Source: CAD feature listing. Evaluate the final solid. Frame: model axes, mm. A direction names the side the tool comes from. Give positions to 0.01 mm unless a question says otherwise; leave off trailing zeros. Loops run counter-clockwise (first coordinate to the right, second up) from the corner with the lowest first, then second, coordinate; pieces in that order, holes last.
```python
from build123d import *

# Parameters (mm, degrees)
SKETCH1_R           = 5.1
SKETCH1_R_2         = 1.25
SKETCH1_R_3         = 1.5
BOSS_EXTRUDE1_DEPTH = 3
FILLET1_R           = 3
CUT_EXTRUDE1_DEPTH  = 10
BOSS_EXTRUDE2_DEPTH = 3
CUT_EXTRUDE2_DEPTH  = 10
FILLET2_R           = 10


with BuildPart() as part:
    # Sketch1 → Boss-Extrude1 (new body)
    with BuildSketch(Plane(origin=(0, 0, 0), x_dir=(1, 0, 0), z_dir=(0, 1, 0))):
        with BuildLine():
            Line((70, 20), (-70, 20))
            ThreePointArc((-70, 20), (-90, 0), (-70, -20))
            Line((-70, -20), (-41, -20))
            Line((-41, -20), (-28.75, -7.75))
            Line((-28.75, -7.75), (-16.5, -20))
            Line((-16.5, -20), (70, -20))
            ThreePointArc((70, -20), (90, 0), (70, 20))
        make_face()
        with Locations(Location((70, 0, 0), (0, 0, 270))):
            Circle(SKETCH1_R, mode=Mode.SUBTRACT)
        with Locations(Location((59.837325142, 4.209517756, 0), (0, 0, 270))):
            Circle(SKETCH1_R_2, mode=Mode.SUBTRACT)
        with Locations(Location((65.790482244, 10.162674858, 0), (0, 0, 270))):
            Circle(SKETCH1_R_2, mode=Mode.SUBTRACT)
        with Locations(Location((74.209517756, 10.162674858, 0), (0, 0, 270))):
            Circle(SKETCH1_R_2, mode=Mode.SUBTRACT)
        with Locations(Location((80.162674858, 4.209517756, 0), (0, 0, 270))):
            Circle(SKETCH1_R_2, mode=Mode.SUBTRACT)
        with Locations(Location((80.162674858, -4.209517756, 0), (0, 0, 270))):
            Circle(SKETCH1_R_2, mode=Mode.SUBTRACT)
        with Locations(Location((74.209517756, -10.162674858, 0), (0, 0, 270))):
            Circle(SKETCH1_R_2, mode=Mode.SUBTRACT)
        with Locations(Location((65.790482244, -10.162674858, 0), (0, 0, 270))):
            Circle(SKETCH1_R_2, mode=Mode.SUBTRACT)
        with Locations(Location((59.837325142, -4.209517756, 0), (0, 0, 270))):
            Circle(SKETCH1_R_2, mode=Mode.SUBTRACT)
        with Locations(Location((-59.837325142, -4.209517756, 0), (0, 0, 90))):
            Circle(SKETCH1_R_2, mode=Mode.SUBTRACT)
        with Locations(Location((-65.790482244, -10.162674858, 0), (0, 0, 90))):
            Circle(SKETCH1_R_2, mode=Mode.SUBTRACT)
        with Locations(Location((-74.209517756, -10.162674858, 0), (0, 0, 90))):
            Circle(SKETCH1_R_2, mode=Mode.SUBTRACT)
        with Locations(Location((-80.162674858, -4.209517756, 0), (0, 0, 90))):
            Circle(SKETCH1_R_2, mode=Mode.SUBTRACT)
        with Locations(Location((-80.162674858, 4.209517756, 0), (0, 0, 90))):
            Circle(SKETCH1_R_2, mode=Mode.SUBTRACT)
        with Locations(Location((-74.209517756, 10.162674858, 0), (0, 0, 90))):
            Circle(SKETCH1_R_2, mode=Mode.SUBTRACT)
        with Locations(Location((-65.790482244, 10.162674858, 0), (0, 0, 90))):
            Circle(SKETCH1_R_2, mode=Mode.SUBTRACT)
        with Locations(Location((-59.837325142, 4.209517756, 0), (0, 0, 90))):
            Circle(SKETCH1_R_2, mode=Mode.SUBTRACT)
        with Locations(Location((-70, 0, 0), (0, 0, 90))):
            Circle(SKETCH1_R, mode=Mode.SUBTRACT)
        with Locations(Location((-35, 0, 0), (0, 0, 270))):
            Circle(SKETCH1_R_3, mode=Mode.SUBTRACT)
        with Locations(Location((-18.029437252, 16.970562748, 0), (0, 0, 270))):
            Circle(SKETCH1_R_3, mode=Mode.SUBTRACT)
    extrude(amount=BOSS_EXTRUDE1_DEPTH)

    # Fillet1
    fillet1_edges = [part.edges().sort_by_distance(p)[0] for p in [
        (-16.5, 1.5, 20),
        (-28.75, 1.5, 7.75),
        (-41, 1.5, 20),
    ]]
    fillet(fillet1_edges, radius=FILLET1_R)

    # Sketch2 → Cut-Extrude1 (cut)
    with BuildSketch(Plane.XZ):
        Polygon((-28.358163655, 9.01834005), (55, 20), (-28.358163655, 26.558419641), align=None)
    extrude(amount=-CUT_EXTRUDE1_DEPTH, mode=Mode.SUBTRACT)

    # Sketch3 → Boss-Extrude2 (add)
    with BuildSketch(Plane.XZ):
        Polygon((-70, -20), (-29.714195297, -26), (60, -20), align=None)
    extrude(amount=-BOSS_EXTRUDE2_DEPTH)

    # Sketch4 → Cut-Extrude2 (cut)
    with BuildSketch(Plane.XZ):
        Polygon((-29.761678485, 9.168369694), (-60, 20), (-60.52961588, 25.578691215), (-29.998372271, 24.401767037), align=None)
    extrude(amount=-CUT_EXTRUDE2_DEPTH, mode=Mode.SUBTRACT)

    # Fillet2
    # the kernel refuses this fillet: 10 mm, written as the material it adds along each edge
    with BuildSketch(Plane(origin=(60, 0, -20), x_dir=(-0.9977710708464071, 0, -0.06672997963445026), z_dir=(0, 1, 0))) as fillet2_piece_1:
        with BuildLine():
            CenterArc((FILLET2_R * 0.0334022154031, -FILLET2_R), FILLET2_R, 90, 3.826189391)
            Line((-FILLET2_R * 0.0333277642314, -FILLET2_R * 0.00222892915359), (0, 0))
            Line((0, 0), (FILLET2_R * 0.0334022154031, 0))
        make_face()
    extrude(amount=3)
    # the kernel refuses this fillet: 10 mm, written as the material it takes off along each edge
    with BuildSketch(Plane(origin=(-29.714195297, -2.693204599, -26), x_dir=(-0.9890902260552777, 0, 0.14731097963804135), z_dir=(0, 1, 0))) as fillet2_2_piece_1:
        with BuildLine():
            CenterArc((FILLET2_R * 0.107728183948, FILLET2_R), FILLET2_R, 257.702684713, 12.297315287)
            Line((-FILLET2_R * 0.105256420594, FILLET2_R * 0.0229444446563), (0, 0))
            Line((0, 0), (FILLET2_R * 0.107728183948, 0))
        make_face()
    extrude(amount=8.386409197, mode=Mode.SUBTRACT)


solid = part.part
```
(1) Section A-A, the plane z = 0. Return the cut outline in (x, y).
A:
outline: (-90, 0) - (-75.1, 0) - (-75.1, 3) - (-90, 3) - close; (-64.9, 0) - (-36.5, 0) - (-36.5, 3) - (-64.9, 3) - close; (-33.5, 0) - (64.9, 0) - (64.9, 3) - (-33.5, 3) - close; (75.1, 0) - (90, 0) - (90, 3) - (75.1, 3) - close
(2) Ray query, line 1 along Z through (x, y) = (64.5, 2.4); line 2 along X through (y, z) = (1, 8.5); line 3 along X through (y, z) = (2.3, 8). Return the intervals inside material, ascending.
A:
line 1: z = -20 to 20
line 2: x = -88.1 to 88.1
line 3: x = -88.33 to 88.33
(3) Section B-B, the plane y = 0.7. Count the separate pieces of the cut face and the enclosed holes in it, then the cut area to 3 significant figures.
A:
separate pieces: 1
enclosed holes: 20
area: 6,350 mm2
(4) First-contact query: pin 1 (3 mm diameter, centred on x = -59.84, z = -4.21, fed in from +Y); pin 2 (1.8 mm diameter, centred on x = -35, z = 0, fed in from +Y); pin 3 (1 mm diameter, centred on y = 0.5, z = -5, fed in from +X). Flat tips, straight axial feed; report the tip coordinate or a pass-through.
A:
pin 1: stops at y = 3
pin 2: passes through
pin 3: stops at x = 89.49
(5) Reachability of faces 1 (the flat face through (-44.67, 1.48, 14.51)), 2 (the cylindrical face through (-75, 1, 1)), 3 (the flat face through (65, 1, -20)) from +Z, -Z, +X, -X, +Y, -Y: full face, straight path, thin tool, end or side. Return the list, or none.
A:
face 1: +Z, +Y, -Y
face 2: +Y, -Y
face 3: -Z, +X, +Y, -Y
(6) Mould query, pull axis X, two halves, no side actions, for faces 4 (the flat face through (-50.66, 1.48, -22.88)), 5 (the cylindrical face through (-19.36, 1.48, -16.28)), 6 (the cylindrical face through (75, 1, -1)), 7 (the flat face through (-65, 1, 20)). Classes: pulls with the +X half, pulls with the -X half, needs draft (parallel to the pull), parting line crosses it, or undercut.
A:
face 4: pulls with the -X half
face 5: undercut
face 6: undercut
face 7: needs draft
(7) Section C-C, the plane x = -35. Return the cut outline in (y, z), then the cut area to 3 significant figures.
A:
outline: (0, -25.21) - (3, -25.21) - (3, -1.5) - (0, -1.5) - close; (0, 1.5) - (3, 1.5) - (3, 11.04) - (0, 11.04) - close
area: 99.8 mm2
